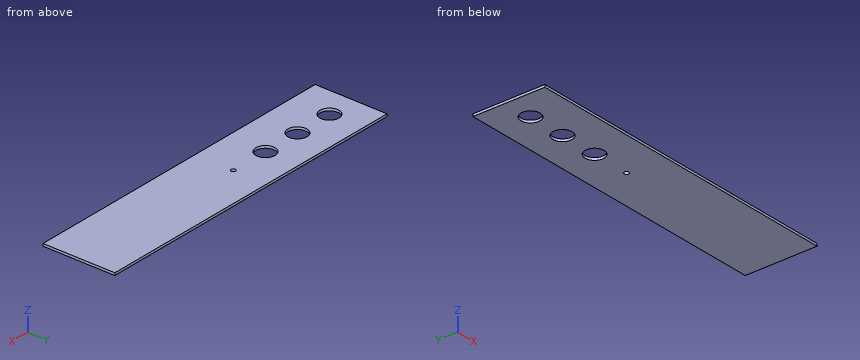
Autodesk Inventor part; units mm, degrees
ref_plane "YZ Plane" through (0, 0, 0) normal (1, 0, 0) x (0, 1, 0)
ref_plane "XZ Plane" through (0, 0, 0) normal (0, 1, 0) x (-1, 0, 0)
ref_plane "XY Plane" through (0, 0, 0) normal (0, 0, 1) x (1, 0, 0)
sketch "Sketch1" plane through (0, 0, 0) normal (0, 0, 1) x (1, 0, 0)
  line L0 (0, 0) -> (431.8, 0)
  line L1 (431.8, 0) -> (431.8, 95.25)
  line L2 (431.8, 95.25) -> (0, 95.25)
  line L3 (0, 95.25) -> (0, 0)
  dimension "d0" = 431.8
  dimension "d1" = 95.25
extrude "Extrusion1" add sketch "Sketch1" along normal blind 3.175
sketch "Sketch2" plane through (0, 0, 3.175) normal (0, 0, 1) x (1, 0, 0)
  line L0 (0, 0) -> (38.1, 0)
  line L1 (0, 50.8) -> (0, 0)
  circle A0 centre (38.1, 50.8) radius 12.7
  circle A1 centre (88.9, 50.8) radius 12.7
  circle A2 centre (139.7, 50.8) radius 12.7
  circle A3 centre (190.5, 50.8) radius 3.048
  dimension "d6" = 25.4
  dimension "d18" = 6.096
extrude "Extrusion2" cut sketch "Sketch2" against normal blind 25.4
properties part number "220207 Front Bottom"
Read the model definition and answer for the solid it produces. Units are mm, in the model's axes. Coordinates: 2 decimals unless noted, no trailing zeros. Write each loop counter-clockwise with the first axis right and the second up, starting at its lowest first coordinate (ties: lowest second). Pieces come first, ordered by that corner, then holes. Notation, with made-up numbers: (8.25, -35.75) -> (24.25, -35.75) arc R26 ccw to (24.25, -20.75) -> close; hole circle Ø6 at (-20.5, 18). An arc over 180 degrees is marked (long way). Return JSON: item names as keys, results as strings.
1. This flat-tipped pin is pushed along its axis until it touches: P1, Ø4, axis at x = 235, y = 65, coming from the -Z side. Where does it stop, or does it pass through?
Found:
{"P1": "z = 0"}
2. A cutting plane is placed at B-B (z = 0.6). Determine the outline of the cut face in (x, y), and give its area (3 significant figures).
Found:
{"outline": "(0, 0) -> (431.8, 0) -> (431.8, 95.25) -> (0, 95.25) -> close; hole circle Ø25.4 at (38.1, 50.8); hole circle Ø25.4 at (88.9, 50.8); hole circle Ø25.4 at (139.7, 50.8); hole circle Ø6.1 at (190.5, 50.8)", "area": "39,600 mm2"}
3. Find the intervals of material crossed by line 1 along X through (y, z) = (52, 2.25); line 2 along Y through (x, z) = (139.7, 2.4); line 3 along X through (y, z) = (53, 2.4), in increasing order. Write a range as from..to.
Found:
{"line 1": "0..25.46, 50.74..76.26, 101.54..127.06, 152.34..187.7, 193.3..431.8", "line 2": "0..38.1, 63.5..95.25", "line 3": "0..25.59, 50.61..76.39, 101.41..127.19, 152.21..188.39, 192.61..431.8"}
4. A cutting plane is placed at C-C (y = 42). Determine the outline of the cut face in (x, z) (3 decimals).
Found:
{"outline": "(0, 0) -> (28.943, 0) -> (28.943, 3.175) -> (0, 3.175) -> close; (47.257, 0) -> (79.743, 0) -> (79.743, 3.175) -> (47.257, 3.175) -> close; (98.057, 0) -> (130.543, 0) -> (130.543, 3.175) -> (98.057, 3.175) -> close; (148.857, 0) -> (431.8, 0) -> (431.8, 3.175) -> (148.857, 3.175) -> close"}
5. A cutting plane is placed at A-A (x = 88.9). Determine the outline of the cut face in (y, z) (3 decimals).
Found:
{"outline": "(0, 0) -> (38.1, 0) -> (38.1, 3.175) -> (0, 3.175) -> close; (63.5, 0) -> (95.25, 0) -> (95.25, 3.175) -> (63.5, 3.175) -> close"}
